Work out the finished part from the listing and answer in its coordinate system (mm). Face numbers are marked on the shaded views. Coordinates: 2 decimals unless noted, no trailing zeros. Loops run counter-clockwise (first coordinate to the right, second up) from the corner with the lowest first, then second, coordinate; pieces in that order, holes last. Notation, with made-up numbers: (-22.5, 24.5) - (22.5, 24.5) arc R28 ccw to (22.5, 61.5) - close; hole circle Ø10 at (87, 39.5). An arc over 180 degrees is marked (long way). Write each question's results on one line, items separated by ' | '. Start each with the question number.
Item 1: Section B-B, the plane z = 18 is taken. Write down the section's boundary in (x, y).
Item 2: Consider probe 1 along X at (y, z) = (0, 13.75); probe 2 along X at (y, z) = (14.5, 14); probe 3 along Y at (x, z) = (2, 8). Determine where each line is inside the solid, lowest interval first. Write a range as [from, to].
Item 3: Section A-A, the plane y = 0 is taken. Write down the section's boundary in (x, z).
Item 4: For a pull along Y with two mould halves and no side action, classify the marked faces 1, 2, 3 and 4 as +Y half, -Y half, draft (parallel to the pull), parting line (faces both ways), or undercut.
Item 5: Section D-D, the plane x = 0 is taken. Write down the section's boundary in (y, z), plus the area to 3 significant figures.
Item 6: Section C-C, the plane y = 11 is taken. Write down the section's boundary in (x, z), plus the area to 3 significant figures.
from build123d import *

# Parameters (mm, degrees)
BOSS_EXTRUDE1_DEPTH = 20


with BuildPart() as part:
    # Sketch1 → Boss-Extrude1 (new body)
    with BuildSketch(Plane.XY):
        with BuildLine():
            Line((-75, 74.379500648), (-75, -15.620499352))
            Line((-75, -15.620499352), (-60, -15.620499352))
            ThreePointArc((-60, -15.620499352), (0, 62), (60, -15.620499352))
            Line((60, -15.620499352), (80, -15.620499352))
            Line((80, -15.620499352), (80, 74.379500648))
            Line((80, 74.379500648), (-75, 74.379500648))
        make_face()
    extrude(amount=BOSS_EXTRUDE1_DEPTH)


solid = part.part
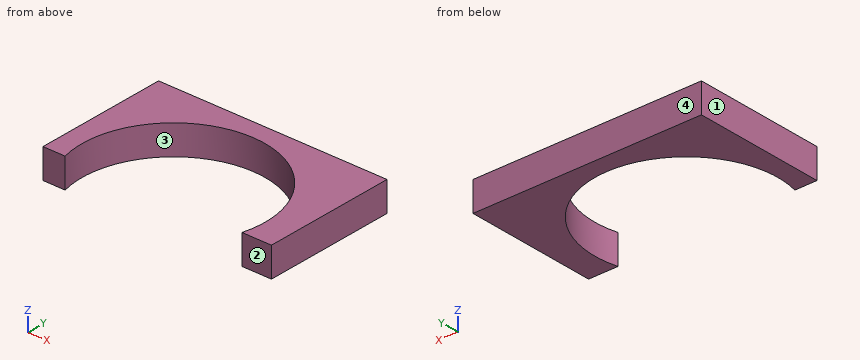
Answer key:
1) outline: (-75, -15.62) - (-60, -15.62) arc R62 cw (long way) to (60, -15.62) - (80, -15.62) - (80, 74.38) - (-75, 74.38) - close
2) probe 1: x = [-75, -62], [62, 80] | probe 2: x = [-75, -60.28], [60.28, 80] | probe 3: y = [61.97, 74.38]
3) outline: (-75, 0) - (-62, 0) - (-62, 20) - (-75, 20) - close; (62, 0) - (80, 0) - (80, 20) - (62, 20) - close
4) face 1: draft | face 2: -Y half | face 3: undercut | face 4: +Y half
5) outline: (62, 0) - (74.38, 0) - (74.38, 20) - (62, 20) - close | area: 248 mm^2
6) outline: (-75, 0) - (-61.02, 0) - (-61.02, 20) - (-75, 20) - close; (61.02, 0) - (80, 0) - (80, 20) - (61.02, 20) - close | area: 659 mm^2
